Geometry: final body of the model. Coordinates: model frame, mm. A direction names the side the tool comes from. Coordinates: 2 decimals unless noted, no trailing zeros. Write each loop counter-clockwise with the first axis right and the second up, starting at its lowest first coordinate (ties: lowest second). Pieces come first, ordered by that corner, then holes. Notation, with made-up numbers: (52, 16.5) -> (96, 16.5) arc R28 ccw to (96, 43.5) -> close; hole circle Ø9 at (-2, -8). An arc over 180 degrees is marked (long way). One line per item, written item: value. Start each with the question number.
Solid Edge part; units mm, degrees
sketch "Sketch1" plane through (0, 0, 0) normal (0, -1, 0) x (1, 0, 0)
  circle A0 centre (0, 0.2989) radius 1.25
  line L0 (-4, 8) -> (-4, 2.2989)
  line L1 (4, 2.2989) -> (4, 8)
  line L2 (4, 8) -> (-4, 8)
  arc A1 (-4, 2.2989) -> (4, 2.2989) centre (0, 2.2989) ccw
  dimension "D1" = 4
  dimension "D2" = 4
extrude "Protrusion1" add sketch "Sketch1" along normal blind 3
sketch "Sketch2" plane through (0, 0, 3.1494) normal (0, 1, 0) x (1, 0, 0)
  circle A0 centre (0, -1.8506) radius 1.25
extrude "ExtrudedProtrusion_2" add sketch "Sketch2" along normal blind 17.5
sketch "Sketch3" plane through (0, 17.5, 5) normal (0, 1, 0) x (0, 0, -1)
  line L0 (-3, -4) -> (6.7011, -4)
  line L1 (6.7011, -4) -> (6.7011, 4)
  line L2 (6.7011, 4) -> (-3, 4)
  line L3 (-3, 4) -> (-3, -4)
extrude "ExtrudedProtrusion_3" add sketch "Sketch3" along normal blind 3
Q1. Access query for faces 4 (the cylindrical face through (-0.27, 8.63, 3.78)), 5 (the flat face through (-4, 19, 3)), 6 (the cylindrical face through (0.1, -1.5, -1.7)). Directions: +Z, -Z, +X, -X, +Y, -Y. A direction counts if a zero-diameter tool reaches every point of the face in a straight line with its end or side. Return the directions, or none.
Q2. Line query: L1, parallel to Y at x = -2, z = 2.25; L2, parallel to Z at x = 0, y = -2.15; L3, parallel to Z at x = 0, y = 12.25. Output: solid intervals per line, ascending. Write a range as from..to.
Q3. Cut plane A-A on x = 0. Output: boundary loops of the cut face in (y, z), and give its area (3 significant figures).
Q4. Draft query along X for faces 1 (the flat face through (4, 19, 3)), 2 (the flat face through (0, -3, 4)), 3 (the cylindrical face through (-0.27, -1.48, 1.52)). Return one class per face: pulls with the +X half, pulls with the -X half, needs draft (parallel to the pull), parting line crosses it, or undercut.
Q5. Cut plane C-C on z = 5. Output: boundary loops of the cut face in (x, y).
Q6. Cut plane D-D on x = -3. Output: boundary loops of the cut face in (y, z), and give its area (3 significant figures).
Q7. Cut plane B-B on z = 7. Output: boundary loops of the cut face in (x, y), and give its area (3 significant figures).
Q8. First-contact query: P1, Ø2, axis at x = -3, y = 0, coming from the -Z side; P2, Ø2, axis at x = 0.5, y = 4, coming from the -Z side; P3, Ø2, axis at x = 0, z = 0.3, coming from the -Y side; P4, Ø1, axis at y = 16.5, z = -0.5, coming from the +X side. Flat tips, straight axial feed; report the tip coordinate or a pass-through.
Solution:
1. face 4: none
1. face 5: +Z, -Z, -X, +Y, -Y
1. face 6: -Z, -Y
2. L1: -3..0, 17.5..20.5
2. L2: -1.7..-0.95, 1.55..8
2. L3: 3.75..6.25
3. outline: (-3, -1.7) -> (0, -1.7) -> (0, -0.95) -> (-3, -0.95) -> close; (-3, 1.55) -> (0, 1.55) -> (0, 3.75) -> (17.5, 3.75) -> (17.5, -1.7) -> (20.5, -1.7) -> (20.5, 8) -> (17.5, 8) -> (17.5, 6.25) -> (0, 6.25) -> (0, 8) -> (-3, 8) -> close
3. area: 94.5 mm²
4. face 1: pulls with the +X half
4. face 2: needs draft
4. face 3: undercut
5. outline: (-4, -3) -> (4, -3) -> (4, 0) -> (1.25, 0) -> (1.25, 17.5) -> (4, 17.5) -> (4, 20.5) -> (-4, 20.5) -> (-4, 17.5) -> (-1.25, 17.5) -> (-1.25, 0) -> (-4, 0) -> close
6. outline: (-3, -0.35) -> (0, -0.35) -> (0, 8) -> (-3, 8) -> close; (17.5, -1.7) -> (20.5, -1.7) -> (20.5, 8) -> (17.5, 8) -> close
6. area: 54.1 mm²
7. outline: (-4, -3) -> (4, -3) -> (4, 0) -> (-4, 0) -> close; (-4, 17.5) -> (4, 17.5) -> (4, 20.5) -> (-4, 20.5) -> close
7. area: 48.0 mm²
8. P1: z = -1.17
8. P2: z = 3.75
8. P3: y = 17.5
8. P4: through
